Input: part model. Units: mm. Frame: model coordinates. A direction names the side the tool comes from. Coordinates: 2 decimals unless noted, no trailing zeros. Write each loop counter-clockwise with the first axis right and the second up, starting at its lowest first coordinate (ties: lowest second). Pieces come first, ordered by that corner, then holes. Notation, with made-up numbers: (-19, 13) - (12, 13) arc R15 ccw to (12, 41) - close; hole circle Ø9 at (-14, -26.5). An arc over 180 degrees is marked (long way). One line per question, with ' | ' between items. Start each with the question number.
1) Section query D-D on x = 12.5. Return loops of the section in (y, z), and give its area (3 significant figures).
2) Reachability of faces 5 (the cylindrical face through (-14.1, -12.57, 3.63)), 6 (the flat face through (-9.37, 13.37, 1.13)) from +Z, -Z, +X, -X, +Y, -Y: full face, straight path, thin tool, end or side. Return the list, or none.
3) Draft query along Y for faces 1 (the flat face through (11.684, -15.646, 1.134)), 2 (the flat face through (13.316, -9.354, 1.134)), 3 (the flat face through (0, 12, 5)), 4 (the flat face through (0, -17.5, 2)). Return one class per face: released by +Y, released by -Y, zero draft, split by the parting line, or undercut.
4) Section query B-B on z = 1.4. Give the number of separate pieces and of enclosed holes in the cut face, and give its area (3 significant figures).
5) Section query A-A on y = 0. Return loops of the section in (x, z), and give its area (3 significant figures).
6) Line query: line 1 (Y direction, x = 12.5, z = 4.3); line 2 (Y direction, x = 0, z = 3.15); line 3 (X direction, y = -14.5, z = 1.5). Output: solid intervals per line, ascending.
7) First-contact query: P1, Ø6, axis at x = -12, y = -12, coming from the -Z side; P2, Ø3.5, axis at x = -12.5, y = 12.5, coming from the -Z side. Flat tips, straight axial feed; report the tip coordinate or a pass-through.
8) Section query C-C on x = 7. Return loops of the section in (y, z), and give its area (3 significant figures).
Autodesk Inventor part; units mm, degrees
ref_plane "YZ Plane" through (0, 0, 0) normal (1, 0, 0) x (0, 1, 0)
ref_plane "XZ Plane" through (0, 0, 0) normal (0, 1, 0) x (-1, 0, 0)
ref_plane "XY Plane" through (0, 0, 0) normal (0, 0, 1) x (1, 0, 0)
sketch "Sketch1" plane through (0, 0, 0) normal (0, 0, 1) x (1, 0, 0)
  circle A0 centre (0, 0) radius 11.5
  circle A1 centre (0, 0) radius 14.3 construction
  line L0 (-17.5, 17.5) -> (17.5, 17.5)
  line L1 (17.5, 17.5) -> (17.5, -17.5)
  line L2 (17.5, -17.5) -> (-17.5, -17.5)
  line L3 (-17.5, -17.5) -> (-17.5, 17.5)
  line L4 (-12.5, 12.5) -> (12.5, 12.5) construction
  line L5 (12.5, 12.5) -> (12.5, -12.5) construction
  line L6 (12.5, -12.5) -> (-12.5, -12.5) construction
  line L7 (-12.5, -12.5) -> (-12.5, 12.5) construction
  line L8 (-9.8464, 15.1536) -> (-8.8751, 11.5287)
  line L9 (-8.8751, 11.5287) -> (-11.5287, 8.8751)
  line L10 (-11.5287, 8.8751) -> (-15.1536, 9.8464)
  line L11 (-15.1536, 9.8464) -> (-16.1249, 13.4713)
  line L12 (-16.1249, 13.4713) -> (-13.4713, 16.1249)
  line L13 (-13.4713, 16.1249) -> (-9.8464, 15.1536)
  line L14 (15.1536, 9.8464) -> (11.5287, 8.8751)
  line L15 (11.5287, 8.8751) -> (8.8751, 11.5287)
  line L16 (8.8751, 11.5287) -> (9.8464, 15.1536)
  line L17 (9.8464, 15.1536) -> (13.4713, 16.1249)
  line L18 (13.4713, 16.1249) -> (16.1249, 13.4713)
  line L19 (16.1249, 13.4713) -> (15.1536, 9.8464)
  line L20 (15.1536, -9.8464) -> (16.1249, -13.4713)
  line L21 (16.1249, -13.4713) -> (13.4713, -16.1249)
  line L22 (13.4713, -16.1249) -> (9.8464, -15.1536)
  line L23 (9.8464, -15.1536) -> (8.8751, -11.5287)
  line L24 (8.8751, -11.5287) -> (11.5287, -8.8751)
  line L25 (11.5287, -8.8751) -> (15.1536, -9.8464)
  line L26 (-15.1536, -9.8464) -> (-11.5287, -8.8751)
  line L27 (-11.5287, -8.8751) -> (-8.8751, -11.5287)
  line L28 (-8.8751, -11.5287) -> (-9.8464, -15.1536)
  line L29 (-9.8464, -15.1536) -> (-13.4713, -16.1249)
  line L30 (-13.4713, -16.1249) -> (-16.1249, -13.4713)
  line L31 (-16.1249, -13.4713) -> (-15.1536, -9.8464)
  line L32 (-12.5, 12.5) -> (12.5, -12.5) construction
  line L33 (12.5, 12.5) -> (-12.5, -12.5) construction
  circle A2 centre (-12.5, 12.5) radius 1.6
  circle A3 centre (12.5, 12.5) radius 1.6
  circle A4 centre (12.5, -12.5) radius 1.6
  circle A5 centre (-12.5, -12.5) radius 1.6
  dimension "d0" = 28.6
  dimension "d1" = 23
  dimension "d6" = 6.5
  dimension "d7" = 25
  dimension "d8" = 25
  dimension "d9" = 3.2
  dimension "d10" = 35
  dimension "d11" = 17.5
  dimension "d12" = 35
  dimension "d13" = 17.5
extrude "Extrusion3" add sketch "Sketch1" along normal blind 5 contours L0 L1 L2 L3 | L8 L9 L10 L11 L12 L13 | L14 L15 L16 L17 L18 L19 | L20 L21 L22 L23 L24 L25 | L26 L27 L28 L29 L30 L31
extrude "Extrusion4" cut sketch "Sketch1" along normal blind 2.3 contours L8 L9 L10 L11 L12 L13 | L14 L15 L16 L17 L18 L19 | L20 L21 L22 L23 L24 L25 | L26 L27 L28 L29 L30 L31
sketch "Sketch2" plane through (0, 0, 5) normal (0, 0, 1) x (1, 0, 0)
  circle A0 centre (-12.5, -12.5) radius 1.6
  circle A1 centre (12.5, -12.5) radius 1.6
  circle A2 centre (12.5, 12.5) radius 1.6
  circle A3 centre (-12.5, 12.5) radius 1.6
  circle A4 centre (0, 0) radius 11.5
  line L0 (17.5, 17.5) -> (-17.5, 17.5)
  line L1 (-17.5, 17.5) -> (-17.5, -17.5)
  line L2 (-17.5, -17.5) -> (17.5, -17.5)
  line L3 (17.5, -17.5) -> (17.5, 17.5)
  dimension "d18" = 23
  dimension "d19" = 12.5
  dimension "d20" = 25
  dimension "d21" = 25
properties part number "BallBearingHolderOutside"
Answer key:
1) outline: (-17.5, 0) - (-15.86, 0) - (-15.86, 2.3) - (-14.1, 2.3) - (-14.1, 5) - (-17.5, 5) - close; (-10.9, 2.3) - (-9.14, 2.3) - (-9.14, 0) - (9.14, 0) - (9.14, 2.3) - (10.9, 2.3) - (10.9, 5) - (-10.9, 5) - close; (14.1, 2.3) - (15.86, 2.3) - (15.86, 0) - (17.5, 0) - (17.5, 5) - (14.1, 5) - close | area: 127 mm²
2) face 5: +Z, -Z | face 6: -Z
3) face 1: undercut | face 2: undercut | face 3: zero draft | face 4: released by -Y
4) separate pieces: 1 | enclosed holes: 5 | area: 663 mm²
5) outline: (-17.5, 0) - (-11.5, 0) - (-11.5, 5) - (-17.5, 5) - close; (11.5, 0) - (17.5, 0) - (17.5, 5) - (11.5, 5) - close | area: 60.0 mm²
6) line 1: -17.5 to -14.1, -10.9 to 10.9, 14.1 to 17.5 | line 2: -17.5 to -11.5, 11.5 to 17.5 | line 3: -17.5 to -15.1, -9.67 to 9.67, 15.1 to 17.5
7) P1: z = 0 | P2: z = 2.3
8) outline: (-17.5, 0) - (-9.12, 0) - (-9.12, 5) - (-17.5, 5) - close; (9.12, 0) - (17.5, 0) - (17.5, 5) - (9.12, 5) - close | area: 83.8 mm²
